Part model, mm, in its own coordinate system. A direction names the side the tool comes from. Round coordinates to 2 decimals unless told otherwise and drop trailing zeros. Write each loop counter-clockwise with the first axis right and the second up, starting at its lowest first coordinate (ties: lowest second). Pieces come first, ordered by that corner, then holes. Notation, with made-up numbers: M 7,66 L 36,66 A25 ccw 36,90 Z; hole C -35.5,17.5 d9. An arc over 180 degrees is marked long. Use one line per item in the form item = value. Start each with the question number.
Item 1: Cut at B-B, the plane x = 9. Give the cut face in (y, z), then the cut area to 3 significant figures.
Item 2: Cut at C-C, the plane z = -219. Give the cut face in (x, y).
Item 3: Cut at A-A, the plane y = 185.5. Give the cut face in (x, z).
Item 4: Which spindle directions (+Z, -Z, +X, -X, +Y, -Y) get a long thin tool onto all of the face, cutting with end or side? Do faces 4 (the face through (20, 100, -2)), 5 (the face through (27, 100, -364)), 6 (the face through (29, 100, -363)), 7 (the face through (38, 100, -14)). Say none if no direction does.
Item 5: Probe L1, parallel to Z at x = 18.5, y = 22.5; L2, parallel to Z at x = 27.5, y = 109; L3, parallel to Y at x = 3, z = -202. List the from-to ranges inside material, lowest first.
Item 6: Mould opens along Z. For faces 1 (the face through (40, 98, -9)), 2 (the face through (20, 99, 0)), 3 (the face through (2, 100, -177)) say: +Z half, -Z half, draft (parallel to the pull), parting line (faces both ways), or undercut.
Item 7: Flat gauge pins, fed straight in: pin 1 Ø12 at (y, z) = (53.5, -365) entering from -X; pin 2 Ø2 at (x, y) = (33, 34.5) entering from -Z; pin 3 Ø1 at (x, y) = (38.5, 105) entering from -Z. Where does each tip first touch, or does it go through?
from build123d import *

# Parameters (mm, degrees)
F4_DEPTH = 2
F6_R     = 2


with BuildPart() as f2:
    # F2: sweep along a path in F1
    with BuildLine(Plane.XY) as f2_path:
        Line((0, 0), (0, 198))
    # F0 (on Front) → F2 (sweep)
    with BuildSketch(Plane.XZ):
        Polygon((40, 0), (0, 0), (0, -350), (27, -350), (27, -376), (29, -376), (29, -348), (2, -348), (2, -2), (38, -2), (38, -25), (40, -25), align=None)
    sweep(path=f2_path.line)


with BuildPart() as f4:
    # F3 (on face) → F4 (new body)
    with BuildSketch(Plane.XZ):
        with BuildLine():
            Line((40, -345), (40, 0))
            Line((40, 0), (0, 0))
            Line((0, 0), (0, -350))
            Line((0, -350), (35, -350))
            ThreePointArc((35, -350), (38.5355339059, -348.5355339059), (40, -345))
        make_face()
    extrude(amount=F4_DEPTH)


with BuildPart() as f2_1:
    add(f2.part)

    # F5: union F4
    add(f4.part)

    # F6
    f6_edges = [f2_1.edges().sort_by_distance(p)[0] for p in [
        (40, 98, 0),
        (0, 98, 0),
        (0, 98, -350),
        (29, 99, -348),
        (27, 99, -350),
        (2, 99, -348),
        (2, 99, -2),
        (38, 99, -2),
    ]]
    fillet(f6_edges, radius=F6_R)


solid = f2_1.part
Model answer:
q1.outline = M -2,-350 L 198,-350 L 198,-348 L 0,-348 L 0,-2 L 198,-2 L 198,0 L -2,0 Z
q1.area = 1,490 mm²
q2.outline = M 0,-2 L 40,-2 L 40,0 L 2,0 L 2,198 L 0,198 Z
q3.outline = M 0,-348 A2 ccw 2,-350 L 25,-350 A2 cw 27,-352 L 27,-376 L 29,-376 L 29,-350 A2 ccw 27,-348 L 4,-348 A2 cw 2,-346 L 2,-4 A2 cw 4,-2 L 36,-2 A2 cw 38,-4 L 38,-25 L 40,-25 L 40,-2 A2 ccw 38,0 L 2,0 A2 ccw 0,-2 Z
q4.face_4 = +Y
q4.face_5 = -Z, -X, +Y, -Y
q4.face_6 = -Z, +X, +Y, -Y
q4.face_7 = -Z, +Y
q5.L1 = -350 to -348, -2 to 0
q5.L2 = -376 to -348.06, -2 to 0
q5.L3 = -2 to 0
q6.face_1 = draft
q6.face_2 = +Z half
q6.face_3 = undercut
q7.pin_1 = 27
q7.pin_2 = -2
q7.pin_3 = -25
